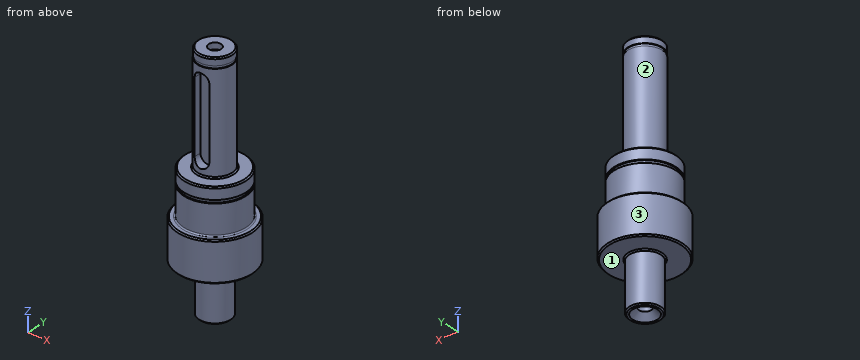
from build123d import *

# Parameters (mm, degrees)
F2_SIZE  = 0.5
F3_R     = 0.5
F6_DEPTH = 3.5


with BuildPart() as f1:
    # F0 (on Front) → F1 (revolve)
    with BuildSketch(Plane.XZ):
        Polygon((0, 15), (0, 0), (0, -68), (2.5, -70.5), (2.5, -75.5), (5, -78), (6.35, -78), (6.35, -58), (15, -58), (15, -42), (12.5, -42), (12.5, -30), (11.95, -30), (11.95, -28.7), (12.475, -28.7), (12.475, -24), (7, -24), (7, 16), (6.7, 16), (6.7, 17.1), (6.975, 17.1), (6.975, 20), (2.5, 20), (2.5, 17.5), align=None)
    revolve(axis=Axis((0, 0, 55.465363), (0, 0, 1)))

    # F2
    f2_edges = [f1.edges().sort_by_distance(p)[0] for p in [
        (-6.975, 0, 20),
        (-12.475, 0, -24),
        (-7, 0, -24),
        (-6.35, 0, -58),
        (-15, 0, -58),
        (-6.35, 0, -78),
        (-15, 0, -42),
    ]]
    chamfer(f2_edges, length=F2_SIZE)

    # F3
    f3_edges = [f1.edges().sort_by_distance(p)[0] for p in [
        (-12.5, 0, -42),
    ]]
    fillet(f3_edges, radius=F3_R)

    # F5 (on offset) → F6 (cut)
    with BuildSketch(Plane.XZ.offset(7)):
        with BuildLine():
            Line((3, -18.5), (3, 10.5))
            ThreePointArc((3, 10.5), (0, 13.5), (-3, 10.5))
            Line((-3, 10.5), (-3, -18.5))
            ThreePointArc((-3, -18.5), (0, -21.5), (3, -18.5))
        make_face()
    extrude(amount=-F6_DEPTH, mode=Mode.SUBTRACT)


solid = f1.part
For this review, take the finished solid that the model builds, in its own axes (mm). Face numbers are marked on the shaded views. A direction names the side the tool comes from. Give positions to 0.01 mm unless a question says otherwise; leave off trailing zeros. Order: outer loops, then holes, each group sorted by start corner. A loop starts at its lowest first (then second) coordinate and runs counter-clockwise, first axis right, second up. Notation, with made-up numbers: (-4, -12.5) -> (5, -12.5) arc R21 ccw to (5, 7.5) -> close; hole circle Ø1 at (9.25, 21). An arc over 180 degrees is marked (long way). Write item = value, one per line.
1) For the marked faces 1, 2 and 3, list the 3-axis set-ups (+Z, -Z, +X, -X, +Y, -Y) from which the entire face can be reached by the end or side of a thin tool; tool diameter is ignored.
Findings:
face_1 = -Z
face_2 = +Z
face_3 = +Z, -Z
2) We need section A-A, the plane z = -50. Give the boundary of the cut face in (x, y), and give its area (3 significant figures).
Findings:
outline = circle Ø30 at (0, 0)
area = 707 mm^2
3) To check wall thickness, follow L1, parallel to Y at x = 0, z = 18.2 (3 decimals); L2, parallel to Y at x = 0, z = -73.3; L3, parallel to Y at x = -1.5, z = -4.5. State the ranges of each line that lie inside material, in increasing order. Write a range as from..to.
Findings:
L1 = -6.975..-2.5, 2.5..6.975
L2 = -6.35..-2.5, 2.5..6.35
L3 = -3.5..6.84
4) We need section C-C, the plane z = 2. Give the boundary of the cut face in (x, y).
Findings:
outline = (-3, -6.32) -> (-3, -3.5) -> (3, -3.5) -> (3, -6.32) arc R7 ccw (long way) to start
5) Insertion check: pin 1 (1.5 mm diameter, centred on y = -2.5, z = -21.5, fed in from +X); pin 2 (2.5 mm diameter, centred on y = -5, z = -5.5, fed in from +X); pin 3 (1.4 mm diameter, centred on y = -4.5, z = -8.5, fed in from -X); pin 4 (1.5 mm diameter, centred on y = -11.5, z = -60, fed in from +X). Each pin has a flat end and moves straight along its axis. Give the tip position at first contact, or say it passes through.
Findings:
pin_1 = 6.78
pin_2 = 5.91
pin_3 = -5.88
pin_4 = through
6) We need section B-B, the plane z = -66. Give the boundary of the cut face in (x, y), and give its area (3 significant figures).
Findings:
outline = circle Ø12.7 at (0, 0)
area = 127 mm^2
